from build123d import *

# Parameters (mm, degrees)
BOSS_EXTRUDE1_DEPTH = 3.175
SKETCH2_R           = 1.524
CUT_EXTRUDE2_DEPTH  = 195.021684248
FILLET1_R           = 12.7
SKETCH3_W           = 12.7
SKETCH3_H           = 3.175
CUT_EXTRUDE3_DEPTH  = 179.341965104
SKETCH4_R           = 1.524
CUT_EXTRUDE4_DEPTH  = 179.341965104


with BuildPart() as part:
    # Sketch1 → Boss-Extrude1 (new body)
    with BuildSketch(Plane(origin=(0, 0, 0), x_dir=(1, 0, 0), z_dir=(0, 1, 0))):
        Polygon((0, 146.646968374), (-127, -73.323484187), (127, -73.323484187), align=None)
    extrude(amount=BOSS_EXTRUDE1_DEPTH)

    # Sketch2 → Cut-Extrude2 (cut, through all)
    with BuildSketch(Plane(origin=(0, 3.175, 0), x_dir=(1, 0, 0), z_dir=(0, 1, 0))):
        with Locations(Location((0, 118.312139176, 0), (0, 0, 270))):
            Circle(SKETCH2_R)
        with Locations(Location((-102.461318102, -59.156069588, 0), (0, 0, 270))):
            Circle(SKETCH2_R)
        with Locations(Location((102.461318102, -59.156069588, 0), (0, 0, 270))):
            Circle(SKETCH2_R)
    extrude(amount=-CUT_EXTRUDE2_DEPTH, mode=Mode.SUBTRACT)

    # Fillet1
    fillet1_edges = [part.edges().sort_by_distance(p)[0] for p in [
        (127, 1.5875, 73.323484187),
        (-127, 1.5875, 73.323484187),
        (0, 1.5875, -146.646968374),
    ]]
    fillet(fillet1_edges, radius=FILLET1_R)

    # Sketch3 → Cut-Extrude3 (cut, through all)
    with BuildSketch(Plane(origin=(0, 3.175, 0), x_dir=(1, 0, 0), z_dir=(0, 1, 0))):
        Polygon((-29.550295474, 90.384355234), (-35.900295474, 79.385832606), (-33.150664817, 77.798332606), (-26.800664817, 88.796855234), align=None)
        Polygon((-83.950664817, -10.189848419), (-86.700295474, -8.602348419), (-93.050295474, -19.600871047), (-90.300664817, -21.188371047), align=None)
        with Locations((-57.15, -69.195984187)):
            Rectangle(SKETCH3_W, SKETCH3_H)
        with Locations((57.15, -69.195984187)):
            Rectangle(SKETCH3_W, SKETCH3_H)
        Polygon((93.050295474, -19.600871047), (86.700295474, -8.602348419), (83.950664817, -10.189848419), (90.300664817, -21.188371047), align=None)
        Polygon((33.150664817, 77.798332606), (35.900295474, 79.385832606), (29.550295474, 90.384355234), (26.800664817, 88.796855234), align=None)
    extrude(amount=-CUT_EXTRUDE3_DEPTH, mode=Mode.SUBTRACT)

    # Sketch4 → Cut-Extrude4 (cut, through all)
    with BuildSketch(Plane(origin=(0, 3.175, 0), x_dir=(1, 0, 0), z_dir=(0, 1, 0))):
        with Locations(Location((-18.034, 69.940515813, 0), (0, 0, 270))):
            Circle(SKETCH4_R)
        with Locations(Location((18.034, 69.940515813, 0), (0, 0, 270))):
            Circle(SKETCH4_R)
        with Locations(Location((-18.034, 11.012515813, 0), (0, 0, 270))):
            Circle(SKETCH4_R)
        with Locations(Location((18.034, 11.012515813, 0), (0, 0, 270))):
            Circle(SKETCH4_R)
    extrude(amount=-CUT_EXTRUDE4_DEPTH, mode=Mode.SUBTRACT)


solid = part.part
Can you work these out from the model? Positions are in its coordinate system, mm. A direction names the side the tool comes from. Give positions to 0.01 mm unless a question says otherwise; leave off trailing zeros. Loops run counter-clockwise (first coordinate to the right, second up) from the corner with the lowest first, then second, coordinate; pieces in that order, holes last. Notation, with made-up numbers: (71, 41) -> (97, 41) arc R31 cw to (97, 65) -> close; hole circle Ø8 at (-6, 30). An arc over 180 degrees is marked (long way). Write item = value, one per line.
1) Suppose I cut it at C-C on y = 0.5. Give the number of separate pieces and of enclosed holes in the cut face, then the cut area to 3 significant figures.
Check result:
separate_pieces = 1
enclosed_holes = 13
area = 27,300 mm2
2) I need wall thicknesses on L1, parallel to X at y = 1.9, z = 11.5; L2, parallel to X at y = 1.75, z = 9; L3, parallel to Z at x = 33.5, y = 2.9. Which ranges of each line are inside material? Lowest first, please. Write a range as from..to.
Check result:
L1 = -91.31..-88.37, -84.71..84.71, 88.37..91.31
L2 = -89.86..-86.93, -86.01..86.01, 86.93..89.86
L3 = -88.62..-83.54, -78..73.32
3) Suppose I cut it at B-B on z = 37. Write out the boundary of the cut face in (x, y) (3 decimals).
Check result:
outline = (-106.029, 0) -> (106.029, 0) -> (106.029, 3.175) -> (-106.029, 3.175) -> close
4) Thinking about a two-plate mould opening in Z: for faces 3 (the flat face through (64.235, 1.565, -35.389)), 4 (the flat face through (-89.83, 1.61, 14.02)), 5 (the cylindrical face through (-116.1, 1.6, 66.8)), which applies, released by +Z, released by -Z, zero draft, split by the parting line, or undercut?
Check result:
face_3 = released by -Z
face_4 = undercut
face_5 = split by the parting line
5) Suppose I cut it at A-A on x = -75. Write out the boundary of the cut face in (y, z) (3 decimals).
Check result:
outline = (0, -16.743) -> (3.175, -16.743) -> (3.175, 73.323) -> (0, 73.323) -> close
6) For faces 1 (the flat face through (-30.02, 1.61, -83.22)), 2 (the flat face through (-62.765, 1.565, -37.935)), which set-ups out of +Z, -Z, +X, -X, +Y, -Y let a thin tool reach every point of the face, with its end or its side?
Check result:
face_1 = +Y, -Y
face_2 = -Z, -X, +Y, -Y
7) Will these pins go through, and if not, where does the flat tip stop? pin 1 (1 mm diameter, centred on y = 2, z = 69, fed in from -X); pin 2 (1 mm diameter, centred on y = 2.5, z = -100, fed in from -X); pin 3 (5 mm diameter, centred on x = 102.46, z = 59.16, fed in from +Y) (3 decimals); pin 4 (1 mm diameter, centred on x = 54.5, y = 2, fed in from -Z).
Check result:
pin_1 = -114.97
pin_2 = -27.22
pin_3 = 3.175
pin_4 = -53.12
